Geometry check sheet. Reference: the model listing, model coordinates, mm. A direction names the side the tool comes from. Coordinates: 2 decimals unless noted, no trailing zeros. Write each loop counter-clockwise with the first axis right and the second up, starting at its lowest first coordinate (ties: lowest second). Pieces come first, ordered by that corner, then holes. Notation, with made-up numbers: (-35.5, 50) -> (4.5, 50) arc R13 ccw to (4.5, 57) -> close; hole circle Ø5 at (74.25, 57). An arc over 180 degrees is marked (long way). Answer in a Markdown table with one row per item. Add a question column.
Q1. Section check D-D, the plane z = 1.5. Record the boundary of the cut face in (x, y) (3 decimals).
Q2. Section check A-A, the plane z = 39.5. Record the boundary of the cut face in (x, y) (3 decimals), and give its area (3 significant figures).
Q3. Thickness scan on line 1 (Y direction, x = 6, z = 53) (3 decimals); line 2 (Z direction, x = 5.5, y = -8); line 3 (Z direction, x = 1.5, y = -17.25). Record the ranges inside material, lowest first.
Q4. Gauge pin test, flat ends, axial feed: P1, Ø4.5, axis at x = 2.5, z = 55.5, coming from the +Y side; P2, Ø2.5, axis at x = 5, z = 59, coming from the +Y side; P3, Ø3, axis at x = 5, y = -11, coming from the +Z side; P4, Ø1.5, axis at y = -12.5, z = 19.5, coming from the +X side. Record the tip position at first contact, or that the pin passes through.
Q5. Release check for a two-part mould opening along Z. For faces 6 (the face through (4, -20.447, 47)), 7 (the face through (4, -22, 51.943)), 8 (the face through (3.882, -16.477, 37.036)) record: pulls with the +Z half, pulls with the -Z half, needs draft (parallel to the pull), parting line crosses it, or undercut.
Q6. Section check B-B, the plane y = -10.25. Record the boundary of the cut face in (x, z), and give its area (3 significant figures).
Q7. Section check C-C, the plane z = 47. Record the boundary of the cut face in (x, y) (3 decimals).
Q8. Tool access check on faces 1 (the face through (3.882, -17.442, 40.048)), 2 (the face through (4, -12.065, 53)), 3 (the face through (3.88, -14.65, 36.33)), 4 (the face through (7.874, -5, 34)), 5 (the face through (3.88, 3.71, -1.35)). Record the directions out of +Z, -Z, +X, -X, +Y, -Y that give a thin tool (end or side, any length) a straight path to the whole face; none if there is none.
```python
from build123d import *

# Parameters (mm, degrees)
F1_DEPTH = 7.874


with BuildPart() as f1:
    # F0 (on Right) → F1 (new body)
    with BuildSketch(Plane.YZ):
        with BuildLine():
            ThreePointArc((2.983524, -1.085914), (-0.551333, -3.126765), (-3.175, 0))
            Line((-3.175, 0), (-3.175, 11.176))
            Line((-3.175, 11.176), (-9.525, 17.526))
            Line((-9.525, 17.526), (-9.525, 26.613775))
            ThreePointArc((-9.525, 26.613775), (-4.870258, 31.466186), (-3.175, 37.973))
            Line((-3.175, 37.973), (-3.175, 57.658))
            ThreePointArc((-3.175, 57.658), (-0.551333, 60.784765), (2.983524, 58.743914))
            Line((2.983524, 58.743914), (4.415616, 59.265153))
            ThreePointArc((4.415616, 59.265153), (-0.815973, 62.285612), (-4.699, 57.658))
            Line((-4.699, 57.658), (-12.065, 57.658))
            Line((-12.065, 57.658), (-12.065, 60.833))
            Line((-12.065, 60.833), (-22.987, 60.833))
            Line((-22.987, 60.833), (-22.987, 51.943))
            Line((-22.987, 51.943), (-20.447, 51.943))
            Line((-20.447, 51.943), (-20.447, 41.783))
            Line((-20.447, 41.783), (-14.351, 38.263473))
            Line((-14.351, 38.263473), (-18.664114, 35.773295))
            Line((-18.664114, 35.773295), (-17.902114, 34.453473))
            Line((-17.902114, 34.453473), (-11.303, 38.263473))
            Line((-11.303, 38.263473), (-18.923, 42.662882))
            Line((-18.923, 42.662882), (-18.923, 53.467))
            Line((-18.923, 53.467), (-21.463, 53.467))
            Line((-21.463, 53.467), (-21.463, 59.309))
            Line((-21.463, 59.309), (-13.589, 59.309))
            Line((-13.589, 59.309), (-13.589, 49.417102))
            ThreePointArc((-13.589, 49.417102), (-4.777528, 39.33271), (-11.049, 27.500312))
            Line((-11.049, 27.500312), (-11.049, 16.894739))
            Line((-11.049, 16.894739), (-4.699, 10.544739))
            Line((-4.699, 10.544739), (-4.699, 0))
            ThreePointArc((-4.699, 0), (-0.815973, -4.627612), (4.415616, -1.607153))
            Line((4.415616, -1.607153), (2.983524, -1.085914))
        make_face()
        with BuildLine():
            Line((-12.065, 56.388), (-4.699, 56.388))
            Line((-4.699, 56.388), (-4.699, 44.163517))
            ThreePointArc((-4.699, 44.163517), (-7.778084, 48.051485), (-12.065, 50.545359))
            Line((-12.065, 50.545359), (-12.065, 56.388))
        make_face(mode=Mode.SUBTRACT)
    extrude(amount=F1_DEPTH)


solid = f1.part
```
Calculated:
| question | item | result |
|---|---|---|
| 1 | outline | (0, -4.699) -> (7.874, -4.699) -> (7.874, -3.175) -> (0, -3.175) -> close |
| 2 | outline | (0, -16.493) -> (7.874, -16.493) -> (7.874, -13.445) -> (0, -13.445) -> close; (0, -4.798) -> (7.874, -4.798) -> (7.874, -3.175) -> (0, -3.175) -> close |
| 2 | area | 36.8 mm² |
| 3 | line 1 | y = -22.987 to -18.923, -13.589 to -12.065, -4.699 to -3.175 |
| 3 | line 2 | z = 13.85 to 16, 27.71 to 29.78, 46.16 to 48.24, 56.39 to 57.66 |
| 3 | line 3 | z = 34.83 to 36.59, 39.94 to 41.7, 59.31 to 60.83 |
| 4 | P1 | stops at y = -3.17 |
| 4 | P2 | stops at y = 4.42 |
| 4 | P3 | stops at z = 60.83 |
| 4 | P4 | passes through |
| 5 | face 6 | needs draft |
| 5 | face 7 | pulls with the -Z half |
| 5 | face 8 | undercut |
| 6 | outline | (0, 16.1) -> (7.87, 16.1) -> (7.87, 27.96) -> (0, 27.96) -> close; (0, 47.99) -> (7.87, 47.99) -> (7.87, 49.75) -> (0, 49.75) -> close; (0, 56.39) -> (7.87, 56.39) -> (7.87, 57.66) -> (0, 57.66) -> close |
| 6 | area | 117 mm² |
| 7 | outline | (0, -20.447) -> (7.874, -20.447) -> (7.874, -18.923) -> (0, -18.923) -> close; (0, -8.893) -> (7.874, -8.893) -> (7.874, -6.695) -> (0, -6.695) -> close; (0, -4.699) -> (7.874, -4.699) -> (7.874, -3.175) -> (0, -3.175) -> close |
| 8 | face 1 | +X, -X, -Y |
| 8 | face 2 | +X, -X |
| 8 | face 3 | -Z, +X, -X |
| 8 | face 4 | +Z, -Z, +X, +Y, -Y |
| 8 | face 5 | +X, -X, +Y |
